The drawing under review shows one solid part. Ordinate dimensions are in mm from its lowest x, y, z. A direction names the side the tool comes from. Round coordinates to 2 decimals unless told otherwise and drop trailing zeros. Write each loop counter-clockwise with the first axis right and the second up, starting at its lowest first coordinate (ties: lowest second). Pieces come first, ordered by that corner, then holes. Notation, with made-up numbers: (23, 30) -> (66, 30) arc R28 ccw to (66, 67) -> close; hole circle Ø2 at (79, 73.5). An arc over 180 degrees is marked (long way). Answer in a Markdown table with one row per item.
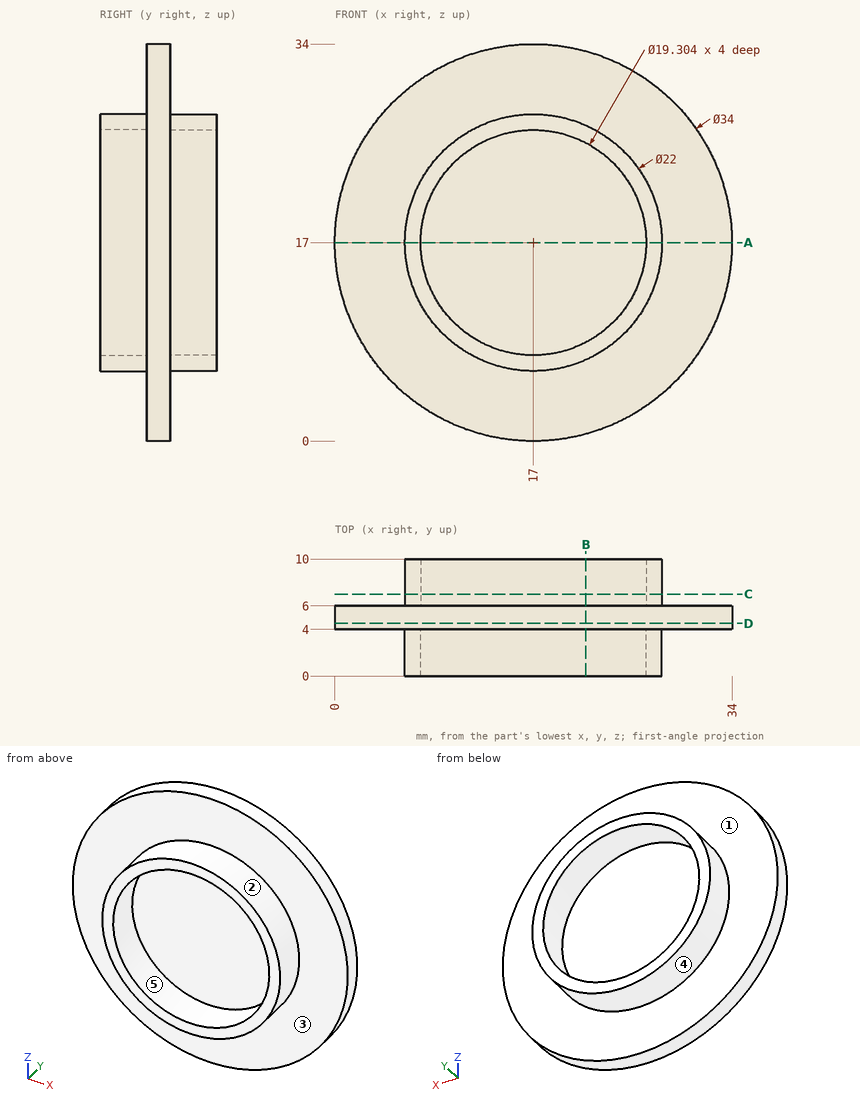
1) Clearance check with flat-ended pins moving along their axes: pin 1 Ø2 at (x, z) = (26.5, 5.5) entering from +Y; pin 2 Ø15.5 at (x, z) = (21.5, 16) entering from +Y; pin 3 Ø15.5 at (x, z) = (18.5, 17) entering from -Y. State where each tip first meets the part, or that it passes through.
Solved:
| item | result |
|---|---|
| pin 1 | y = 6 |
| pin 2 | y = 10 |
| pin 3 | y = 4 |
2) Consider section B-B on x = 21.5. State the section outline as (y, z) points.
Solved:
| item | result |
|---|---|
| outline | (0, 6.96) -> (4, 6.96) -> (4, 0.61) -> (6, 0.61) -> (6, 6.96) -> (10, 6.96) -> (10, 8.46) -> (6, 8.46) -> (6, 25.54) -> (10, 25.54) -> (10, 27.04) -> (6, 27.04) -> (6, 33.39) -> (4, 33.39) -> (4, 27.04) -> (0, 27.04) -> (0, 25.54) -> (4, 25.54) -> (4, 8.46) -> (0, 8.46) -> close |
3) Consider section C-C on y = 7. State the section outline as (x, z) points.
Solved:
| item | result |
|---|---|
| outline | circle Ø22 at (17, 17); hole circle Ø19.3 at (17, 17) |
4) Consider section A-A on z = 17. State the section outline as (x, y) points, then the cut area to 3 significant figures.
Solved:
| item | result |
|---|---|
| outline | (0, 4) -> (6, 4) -> (6, 0) -> (7.35, 0) -> (7.35, 4) -> (26.65, 4) -> (26.65, 0) -> (28, 0) -> (28, 4) -> (34, 4) -> (34, 6) -> (28, 6) -> (28, 10) -> (26.65, 10) -> (26.65, 6) -> (7.35, 6) -> (7.35, 10) -> (6, 10) -> (6, 6) -> (0, 6) -> close |
| area | 89.6 mm² |
5) For the marked faces 1 and 2, list the 3-axis set-ups (+Z, -Z, +X, -X, +Y, -Y) from which the entire face can be reached by the end or side of a thin tool; tool diameter is ignored.
Solved:
| item | result |
|---|---|
| face 1 | +Y |
| face 2 | -Y |
6) Consider section D-D on y = 4.5. State the section outline as (x, z) points.
Solved:
| item | result |
|---|---|
| outline | circle Ø34 at (17, 17) |
7) For line 1 (X direction, y = 2.05, z = 17); line 2 (Y direction, x = 27, z = 29); line 3 (X direction, y = 3.75, z = 20.5), list the stretches that pass through material, from the lowest coordinate up. Write a range as [from, to].
Solved:
| item | result |
|---|---|
| line 1 | [6, 7.35], [26.65, 28] |
| line 2 | [4, 6] |
| line 3 | [6.57, 8], [26, 27.43] |
8) Mouldability with a two-part tool opening along X and no side actions: class the marked faces 3, 4 and 5 as pulls with the +X half, pulls with the -X half, needs draft (parallel to the pull), parting line crosses it, or undercut.
Solved:
| item | result |
|---|---|
| face 3 | needs draft |
| face 4 | parting line crosses it |
| face 5 | undercut |
